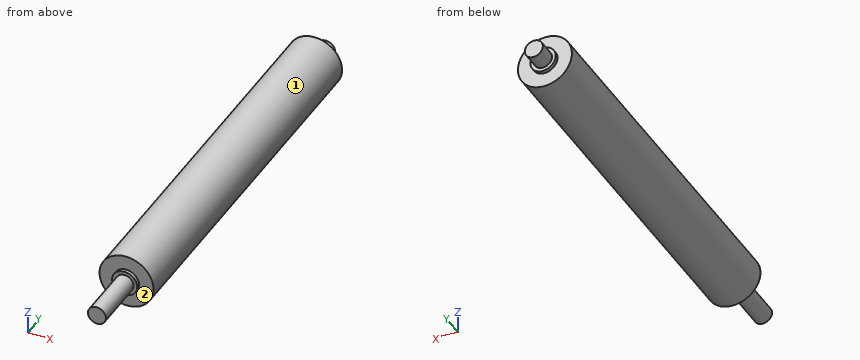
from build123d import *

# Parameters (mm, degrees)
SKETCH1_R           = 7.5
BOSS_EXTRUDE1_DEPTH = 102
SKETCH2_R           = 3.5
BOSS_EXTRUDE2_DEPTH = 1
SKETCH3_R           = 2.5
BOSS_EXTRUDE3_DEPTH = 15
BOSS_EXTRUDE4_START = 1
SKETCH4_R           = 3.5
BOSS_EXTRUDE4_DEPTH = 1
BOSS_EXTRUDE5_START = 5
SKETCH5_R           = 2.5
BOSS_EXTRUDE5_DEPTH = 5


with BuildPart() as part:
    # Sketch1 → Boss-Extrude1 (new body)
    with BuildSketch(Plane(origin=(0, 0, 0), x_dir=(1, 0, 0), z_dir=(0, 1, 0))):
        with Locations(Location((0, 0, 0), (0, 0, 270))):
            Circle(SKETCH1_R)
    extrude(amount=BOSS_EXTRUDE1_DEPTH)

    # Sketch2 → Boss-Extrude2 (add)
    with BuildSketch(Plane.XZ):
        with Locations(Location((0, 0, 0), (0, 0, 270))):
            Circle(SKETCH2_R)
    extrude(amount=BOSS_EXTRUDE2_DEPTH)

    # Sketch3 → Boss-Extrude3 (add)
    with BuildSketch(Plane.XZ.offset(1)):
        with Locations(Location((0, 0, 0), (0, 0, 270))):
            Circle(SKETCH3_R)
    extrude(amount=BOSS_EXTRUDE3_DEPTH)

    # Sketch4 → Boss-Extrude4 (add)
    with BuildSketch(Plane(origin=(0, 102, 0), x_dir=(1, 0, 0), z_dir=(0, 1, 0)).offset(BOSS_EXTRUDE4_START)):
        with Locations(Location((0, 0, 0), (0, 0, 90))):
            Circle(SKETCH4_R)
    extrude(amount=-BOSS_EXTRUDE4_DEPTH)

    # Sketch5 → Boss-Extrude5 (add)
    with BuildSketch(Plane(origin=(0, 103, 0), x_dir=(1, 0, 0), z_dir=(0, 1, 0)).offset(BOSS_EXTRUDE5_START)):
        with Locations(Location((0, 0, 0), (0, 0, 90))):
            Circle(SKETCH5_R)
    extrude(amount=-BOSS_EXTRUDE5_DEPTH)


solid = part.part
Work out the finished part from the listing and answer in its coordinate system (mm). Face numbers are marked on the shaded views. A direction names the side the tool comes from. Coordinates: 2 decimals unless noted, no trailing zeros. Loops run counter-clockwise (first coordinate to the right, second up) from the corner with the lowest first, then second, coordinate; pieces in that order, holes last. Notation, with made-up numbers: (44, -40) -> (90, -40) arc R35 ccw to (90, -2) -> close; hole circle Ø3 at (74, 63.25). An arc over 180 degrees is marked (long way). Write each question's results on one line, items separated by ' | '. Start each with the question number.
1) Find section B-B on x = 0. Determine the outline of the cut face in (y, z).
2) Find section C-C on y = 51.5. Determine the outline of the cut face in (x, z), then the cut area to 3 significant figures.
3) Find section A-A on z = 0. Determine the outline of the cut face in (x, y).
4) Find section D-D on z = 5.75. Determine the outline of the cut face in (x, y).
5) Consider line 1 along Y through (x, z) = (4, 1.75); line 2 along Y through (x, z) = (1.25, -2.25); line 3 along Z through (x, y) = (-2.75, 37). Determine where each line is inside the solid, lowest interval first.
6) Flat-ended cylindrical pins translate along their axes: P1, Ø3, axis at x = -3.5, z = -3.5, coming from the -Y side; P2, Ø1.5, axis at y = 32, z = -3, coming from the -X side; P3, Ø2, axis at y = 5, z = -4, coming from the -X side. Find the tip coordinate at first contact, or state that the pin passes through.
7) For the marked faces 1 and 2, determine the directions among +Z, -Z, +X, -X, +Y, -Y from which every point of the face is accessible in a straight line to the end or side of a thin tool.
Response values:
1) outline: (-16, -2.5) -> (-1, -2.5) -> (-1, -3.5) -> (0, -3.5) -> (0, -7.5) -> (102, -7.5) -> (102, -3.5) -> (103, -3.5) -> (103, -2.5) -> (108, -2.5) -> (108, 2.5) -> (103, 2.5) -> (103, 3.5) -> (102, 3.5) -> (102, 7.5) -> (0, 7.5) -> (0, 3.5) -> (-1, 3.5) -> (-1, 2.5) -> (-16, 2.5) -> close
2) outline: circle Ø15 at (0, 0) | area: 177 mm^2
3) outline: (-7.5, 0) -> (-3.5, 0) -> (-3.5, -1) -> (-2.5, -1) -> (-2.5, -16) -> (2.5, -16) -> (2.5, -1) -> (3.5, -1) -> (3.5, 0) -> (7.5, 0) -> (7.5, 102) -> (3.5, 102) -> (3.5, 103) -> (2.5, 103) -> (2.5, 108) -> (-2.5, 108) -> (-2.5, 103) -> (-3.5, 103) -> (-3.5, 102) -> (-7.5, 102) -> close
4) outline: (-4.82, 0) -> (4.82, 0) -> (4.82, 102) -> (-4.82, 102) -> close
5) line 1: y = 0 to 102 | line 2: y = -1 to 103 | line 3: z = -6.98 to 6.98
6) P1: stops at y = -1 | P2: stops at x = -7.15 | P3: stops at x = -6.87
7) face 1: +Y, -Y | face 2: -Y
